```python
from build123d import *

# Parameters (mm, degrees)
SKETCH2_W               = 114.3
SKETCH2_H               = 101.6
BOSS_EXTRUDE1_DEPTH     = 2.54
SKETCH3_W               = 19.05
SKETCH3_H               = 38.1
BOSS_EXTRUDE2_DEPTH     = 2.54
TRUCKMOUNTINGHOLES_R    = 2.38125
CUT_EXTRUDE1_DEPTH      = 6.08
FILLET1_R               = 2.54
CUT_EXTRUDE3_DEPTH      = 3.54
CUT_EXTRUDE3_DEPTH_BACK = 3.54
BOSS_EXTRUDE3_DEPTH     = 2.54
CUT_EXTRUDE4_DEPTH      = 1.525958
FILLET2_R               = 6.35
SKETCH8_W               = 22.225
SKETCH8_H               = 2.54
BOSS_EXTRUDE4_DEPTH     = 2.54
CUT_EXTRUDE5_DEPTH      = 2.54
SKETCH10_W              = 60.325
SKETCH10_H              = 101.6
CUT_EXTRUDE6_DEPTH      = 2.54


with BuildPart() as part:
    # Sketch2 → Boss-Extrude1 (new body)
    with BuildSketch(Plane(origin=(0, 0, 0), x_dir=(1, 0, 0), z_dir=(0, 1, 0))):
        Rectangle(SKETCH2_W, SKETCH2_H)
    extrude(amount=BOSS_EXTRUDE1_DEPTH)

    # Sketch3 → Boss-Extrude2 (add)
    with BuildSketch(Plane(origin=(0, 2.54, 0), x_dir=(1, 0, 0), z_dir=(0, 1, 0))):
        with Locations((-20.6375, -31.75)):
            Rectangle(SKETCH3_W, SKETCH3_H)
        with Locations((20.6375, -31.75)):
            Rectangle(SKETCH3_W, SKETCH3_H)
        Polygon((-30.1625, 41.705647627), (-30.1625, 12.7), (-11.1125, 12.7), (-11.1125, 50.8), (-23.794565913, 50.8), align=None)
        Polygon((11.1125, 50.8), (11.1125, 12.7), (30.1625, 12.7), (30.1625, 41.705647627), (23.794565913, 50.8), align=None)
    extrude(amount=BOSS_EXTRUDE2_DEPTH)

    # TruckMountingHoles → Cut-Extrude1 (cut, through all)
    with BuildSketch(Plane(origin=(0, 0, 0), x_dir=(1, 0, 0), z_dir=(0, 1, 0))):
        with Locations((-20.6375, 22.225)):
            Circle(TRUCKMOUNTINGHOLES_R)
        with Locations((-20.6375, 31.75)):
            Circle(TRUCKMOUNTINGHOLES_R)
        with Locations((20.6375, 31.75)):
            Circle(TRUCKMOUNTINGHOLES_R)
        with Locations((20.6375, 22.225)):
            Circle(TRUCKMOUNTINGHOLES_R)
        with Locations((20.6375, -31.75)):
            Circle(TRUCKMOUNTINGHOLES_R)
        with Locations((-20.6375, -31.75)):
            Circle(TRUCKMOUNTINGHOLES_R)
    extrude(amount=CUT_EXTRUDE1_DEPTH, mode=Mode.SUBTRACT)

    # Fillet1
    fillet1_edges = [part.edges().sort_by_distance(p)[0] for p in [
        (57.15, 1.27, 50.8),
        (-57.15, 1.27, 50.8),
        (-57.15, 1.27, -50.8),
        (57.15, 1.27, -50.8),
    ]]
    fillet(fillet1_edges, radius=FILLET1_R)

    # Sketch5 → Cut-Extrude3 (cut, two sides)
    with BuildSketch(Plane(origin=(0, 2.54, 0), x_dir=(1, 0, 0), z_dir=(0, 1, 0))) as cut_extrude3_sk:
        with BuildLine():
            Line((54.61, 50.8), (36.197635735, 50.8))
            Line((36.197635735, 50.8), (57.15, 20.876922739))
            Line((57.15, 20.876922739), (57.15, 48.26))
            ThreePointArc((57.15, 48.26), (56.406051224, 50.056051224), (54.61, 50.8))
        make_face()
        with BuildLine():
            Line((-57.15, 20.876922739), (-36.197635735, 50.8))
            Line((-36.197635735, 50.8), (-54.61, 50.8))
            ThreePointArc((-54.61, 50.8), (-56.406051224, 50.056051224), (-57.15, 48.26))
            Line((-57.15, 48.26), (-57.15, 20.876922739))
        make_face()
    extrude(amount=CUT_EXTRUDE3_DEPTH, mode=Mode.SUBTRACT)
    extrude(cut_extrude3_sk.sketch, amount=-CUT_EXTRUDE3_DEPTH_BACK, mode=Mode.SUBTRACT)

    # Sketch5<5> → Boss-Extrude3 (add)
    with BuildSketch(Plane(origin=(0, 2.54, 0), x_dir=(1, 0, 0), z_dir=(0, 1, 0))):
        Polygon((36.197635735, 50.8), (27.305, 63.5), (-27.305, 63.5), (-36.197635735, 50.8), (-25.500724295, 50.8), (-23.794565913, 50.8), (-11.1125, 50.8), (11.1125, 50.8), (23.794565913, 50.8), align=None)
    extrude(amount=-BOSS_EXTRUDE3_DEPTH)

    # Sketch6 → Cut-Extrude4 (cut)
    with BuildSketch(Plane(origin=(0, 2.54, 0), x_dir=(1, 0, 0), z_dir=(0, 1, 0))):
        with BuildLine():
            Line((49.383451528, 23.776246966), (52.400388507, 25.888728981))
            Line((52.400388507, 25.888728981), (28.747959175, 59.667898786))
            ThreePointArc((28.747959175, 59.667898786), (26.387666917, 61.737819542), (23.338279075, 62.484))
            Line((23.338279075, 62.484), (-23.338279075, 62.484))
            ThreePointArc((-23.338279075, 62.484), (-26.387666917, 61.737819542), (-28.747959175, 59.667898786))
            Line((-28.747959175, 59.667898786), (-52.400388507, 25.888728981))
            Line((-52.400388507, 25.888728981), (-49.383451528, 23.776246966))
            Line((-49.383451528, 23.776246966), (-25.731022196, 57.555416771))
            ThreePointArc((-25.731022196, 57.555416771), (-24.687046774, 58.470958644), (-23.338279075, 58.801))
            Line((-23.338279075, 58.801), (23.338279075, 58.801))
            ThreePointArc((23.338279075, 58.801), (24.687046774, 58.470958644), (25.731022196, 57.555416771))
            Line((25.731022196, 57.555416771), (49.383451528, 23.776246966))
        make_face()
    extrude(amount=-CUT_EXTRUDE4_DEPTH, mode=Mode.SUBTRACT)

    # Fillet2
    fillet2_edges = [part.edges().sort_by_distance(p)[0] for p in [
        (57.15, 1.27, -20.876922739),
        (-57.15, 1.27, -20.876922739),
        (-27.305, 1.27, -63.5),
        (27.305, 1.27, -63.5),
    ]]
    fillet(fillet2_edges, radius=FILLET2_R)

    # Sketch8 → Boss-Extrude4 (add)
    with BuildSketch(Plane(origin=(0, 2.54, 0), x_dir=(1, 0, 0), z_dir=(0, 1, 0))):
        with Locations((0, -49.53)):
            Rectangle(SKETCH8_W, SKETCH8_H)
    extrude(amount=BOSS_EXTRUDE4_DEPTH)

    # Sketch9 → Cut-Extrude5 (cut)
    with BuildSketch(Plane.XY.offset(50.8)):
        with BuildLine():
            Line((6.346056871, 5.08), (-6.346056871, 5.08))
            ThreePointArc((-6.346056871, 5.08), (-5.941945474, 4.247288898), (-5.08, 3.91))
            Line((-5.08, 3.91), (5.08, 3.91))
            ThreePointArc((5.08, 3.91), (5.941945474, 4.247288898), (6.346056871, 5.08))
        make_face()
    extrude(amount=-CUT_EXTRUDE5_DEPTH, mode=Mode.SUBTRACT)

    # Sketch10 → Cut-Extrude6 (cut)
    with BuildSketch(Plane(origin=(0, 5.08, 0), x_dir=(1, 0, 0), z_dir=(0, 1, 0))):
        Rectangle(SKETCH10_W, SKETCH10_H)
    extrude(amount=-CUT_EXTRUDE6_DEPTH, mode=Mode.SUBTRACT)


solid = part.part
```
Verification items for the finished model (mm, model axes). A direction names the side the tool comes from. Give positions to 0.01 mm unless a question says otherwise; leave off trailing zeros. Loops run counter-clockwise (first coordinate to the right, second up) from the corner with the lowest first, then second, coordinate; pieces in that order, holes last.
1. Section check D-D, the plane z = -40. Enter the section's corners in (x, y).
2. Set-up check for faces 1 (the flat face through (37.392, 1.788, -40.902)), 2 (the cylindrical face through (-56.426, 1.288, 50.036)): record each of +Z, -Z, +X, -X, +Y, -Y from which the full face is reachable in a straight line by a thin tool's end or side.
3. Section check B-B, the plane y = 1.75. Count the separate pieces of the cut face and the enclosed holes in it, then the cut area to 3 significant figures.
4. Mould release check, pull along X, two halves, no side actions. Record for faces 3 (the flat face through (-57.15, 1, 15)), 4 (the flat face through (57.15, 1, 15)), 5 (the flat face through (40.74, 1.79, -42.54)), 6 (the flat face through (0, 1, -63.5)): released by +X, released by -X, zero draft, split by the parting line, or undercut.
5. Section check C-C, the plane x = 40. Enter the section's corners in (y, z).
6. Go/stop test with a flat-tipped pin: pin 1 Ø4.5 at (x, z) = (-20.64, -22.22) entering from -Y. Record where the tip stops, or that it passes through.
7. Thickness scan on line 1 (X direction, y = 1.9, z = -31.75); line 2 (X direction, y = 2.35, z = -50.5); line 3 (X direction, y = 0.8, z = 31). Record the ranges inside material, lowest first.
8. Section check A-A, the plane z = 31.75. Enter the section's corners in (x, y), then the cut area to 3 significant figures.
Geometry says:
1. outline: (-43.76, 0) - (43.76, 0) - (43.76, 2.54) - (42.52, 2.54) - (42.52, 1.01) - (38.02, 1.01) - (38.02, 2.54) - (-38.02, 2.54) - (-38.02, 1.01) - (-42.52, 1.01) - (-42.52, 2.54) - (-43.76, 2.54) - close
2. face 1: +Y
2. face 2: +Z, -X, +Y, -Y
3. separate pieces: 1
3. enclosed holes: 7
3. area: 11,200 mm2
4. face 3: released by -X
4. face 4: released by +X
4. face 5: undercut
4. face 6: zero draft
5. outline: (0, -45.37) - (2.54, -45.37) - (2.54, -43.6) - (1.01, -43.6) - (1.01, -37.18) - (2.54, -37.18) - (2.54, 50.8) - (0, 50.8) - close
6. pin 1: passes through
7. line 1: x = -49.54 to -48.3, -43.8 to -23.02, -18.26 to 18.26, 23.02 to 43.8, 48.3 to 49.54
7. line 2: x = -36.41 to -35.17, -30.67 to 30.67, 35.17 to 36.41
7. line 3: x = -57.15 to -22.9, -18.38 to 18.38, 22.9 to 57.15
8. outline: (-57.15, 0) - (-23.02, 0) - (-23.02, 2.54) - (-57.15, 2.54) - close; (-18.26, 0) - (18.26, 0) - (18.26, 2.54) - (-18.26, 2.54) - close; (23.02, 0) - (57.15, 0) - (57.15, 2.54) - (23.02, 2.54) - close
8. area: 266 mm2
